Here's how the part is built. I have some questions about the finished solid (model axes, mm). A direction names the side the tool comes from. Give positions to 0.01 mm unless a question says otherwise; leave off trailing zeros. Loops run counter-clockwise (first coordinate to the right, second up) from the corner with the lowest first, then second, coordinate; pieces in that order, holes last.
Q1. If we section it at A-A (z = 8.5): Please give me the cut outline in (x, y), plus the area to 3 significant figures.
Q2. If we section it at D-D (y = 48): Please give me the cut outline in (x, z).
Q3. If we section it at C-C (x = 26.5): Please give me the cut outline in (y, z).
Q4. For faces 1 (the face through (45, 40, 5)), 2 (the face through (-1, 25, 15)), 3 (the face through (20.246, 19.152, 7.042)), which set-ups out of +Z, -Z, +X, -X, +Y, -Y let a thin tool reach every point of the face, with its end or its side?
Q5. I need wall thicknesses on line 1 (X direction, y = 72, z = 13.25); line 2 (Z direction, x = 18, y = 73.5); line 3 (Z direction, x = 13, y = 15.5). Which ranges of each line are inside material? Lowest first, please.
Q6. Will these pins go through, and if not, where does the flat tip stop? P1, Ø3, axis at x = 31.5, z = 8.5, coming from the +Y side; P2, Ø1.5, axis at x = 36.5, z = 5.5, coming from the -Y side; P3, Ø0.9, axis at x = -2, y = 62.5, coming from the -Z side; P4, Ø15, axis at y = 49.5, z = 16, coming from the -X side.
Q7. If we section it at B-B (y = 17.5): Please give me the cut outline in (x, z).
Q8. We'd pull the mould along Y, two halves only. Please class faces 4 (the face through (-1, 10, 15)), 5 (the face through (-1, 18, 18)), 6 (the face through (2.465, 42.747, 15.121)), 7 (the face through (27.695, 15.563, 4.93)): +Y half, -Y half, draft (parallel to the pull), parting line (faces both ways), or undercut.
from build123d import *

# Parameters (mm, degrees)
PAD_DEPTH       = 10
SKETCH001_R     = 2
POCKET_DEPTH    = 10.001
SKETCH002_R     = 5.5
POCKET001_DEPTH = 6
SKETCH004_W     = 5
SKETCH004_H     = 80
PAD001_DEPTH    = 20
SKETCH006_W     = 15
SKETCH006_H     = 6
PAD002_DEPTH    = 3
POCKET004_DEPTH = 10.001
SKETCH008_R     = 2.75
POCKET005_DEPTH = 55.001
FILLET_R        = 5
FILLET001_R     = 1


with BuildPart() as part:
    # Sketch → Pad (new body)
    with BuildSketch(Plane.XY):
        with BuildLine():
            Line((0, 0), (0, 80))
            Line((0, 80), (15, 80))
            ThreePointArc((15, 0), (55, 40), (15, 80))
            Line((0, 0), (15, 0))
        make_face()
    extrude(amount=PAD_DEPTH)

    # Sketch001 (on Face6 of Pad) → Pocket (cut, through all)
    with BuildSketch(Plane.XY.offset(10)):
        with Locations((15, 62.5)):
            Circle(SKETCH001_R)
        with Locations((15, 17.5)):
            Circle(SKETCH001_R)
    extrude(amount=-POCKET_DEPTH, mode=Mode.SUBTRACT)

    # Sketch002 (on Face5 of Pocket) → Pocket001 (cut)
    with BuildSketch(Plane.XY.offset(10)):
        with Locations((15, 62.5)):
            Circle(SKETCH002_R)
        with Locations((15, 17.5)):
            Circle(SKETCH002_R)
    extrude(amount=-POCKET001_DEPTH, mode=Mode.SUBTRACT)

    # Sketch004 → Pad001 (join)
    with BuildSketch(Plane.XY.offset(10)):
        with Locations((2.5, 40)):
            Rectangle(SKETCH004_W, SKETCH004_H)
    extrude(amount=PAD001_DEPTH)

    # Sketch006 → Pad002 (join)
    with BuildSketch(Plane(origin=(0, 0, 0), x_dir=(0, -1, 0), z_dir=(-1, 0, 0))):
        with Locations((-62.5, 15)):
            Rectangle(SKETCH006_W, SKETCH006_H)
        with Locations((-17.5, 15)):
            Rectangle(SKETCH006_W, SKETCH006_H)
    extrude(amount=PAD002_DEPTH)

    # Sketch007 (on Face8 of Pad002) → Pocket004 (cut, through all)
    with BuildSketch(Plane.XY.offset(10)):
        with BuildLine():
            ThreePointArc((25, 11.715729), (45, 40), (25, 68.284271))
            Line((25, 68.284271), (25, 11.715729))
        make_face()
    extrude(amount=-POCKET004_DEPTH, mode=Mode.SUBTRACT)

    # Sketch008 (on Face5 of Pocket004) → Pocket005 (cut, through all)
    with BuildSketch(Plane(origin=(0, 0, 0), x_dir=(0, -1, 0), z_dir=(-1, 0, 0))):
        with Locations((-40, 15)):
            Circle(SKETCH008_R)
    extrude(amount=-POCKET005_DEPTH, mode=Mode.SUBTRACT)

    # Fillet
    fillet_edges = [part.edges().sort_by_distance(p)[0] for p in [
        (25, 68.284271, 5),
        (25, 11.715729, 5),
    ]]
    fillet(fillet_edges, radius=FILLET_R)

    # Fillet001
    fillet001_edges = [part.edges().sort_by_distance(p)[0] for p in [
        (5, 40, 10),
    ]]
    fillet(fillet001_edges, radius=FILLET001_R)


solid = part.part
Check sheet entries:
1. outline: (0, 0) - (15, 0) arc R40 ccw to (15, 80) - (0, 80) - close; hole circle Ø11 at (15, 17.5); hole circle Ø11 at (15, 62.5); hole (25, 20) arc R5 ccw to (33, 16) arc R30 ccw to (33, 64) arc R5 ccw to (25, 60) - close
1. area: 2,730 mm2
2. outline: (0, 0) - (25, 0) - (25, 10) - (6, 10) arc R1 cw to (5, 11) - (5, 30) - (0, 30) - close; (43.91, 0) - (54.19, 0) - (54.19, 10) - (43.91, 10) - close
3. outline: (1.69, 0) - (16.43, 0) - (16.43, 10) - (1.69, 10) - close; (63.57, 0) - (78.31, 0) - (78.31, 10) - (63.57, 10) - close
4. face 1: +Z, -Z
4. face 2: +Z, -Z, -X
4. face 3: +Z
5. line 1: x = 0 to 5
5. line 2: z = 0 to 10
5. line 3: z = 0 to 4
6. P1: stops at y = 77.08
6. P2: stops at y = 5.8
6. P3: stops at z = 12
6. P4: stops at x = -3
7. outline: (-3, 12) - (0, 12) - (0, 0) - (13, 0) - (13, 4) - (9.5, 4) - (9.5, 10) - (6, 10) arc R1 cw to (5, 11) - (5, 30) - (0, 30) - (0, 18) - (-3, 18) - close; (17, 0) - (25.67, 0) - (25.67, 10) - (20.5, 10) - (20.5, 4) - (17, 4) - close; (34.84, 0) - (48.07, 0) - (48.07, 10) - (34.84, 10) - close
8. face 4: -Y half
8. face 5: draft
8. face 6: undercut
8. face 7: undercut
